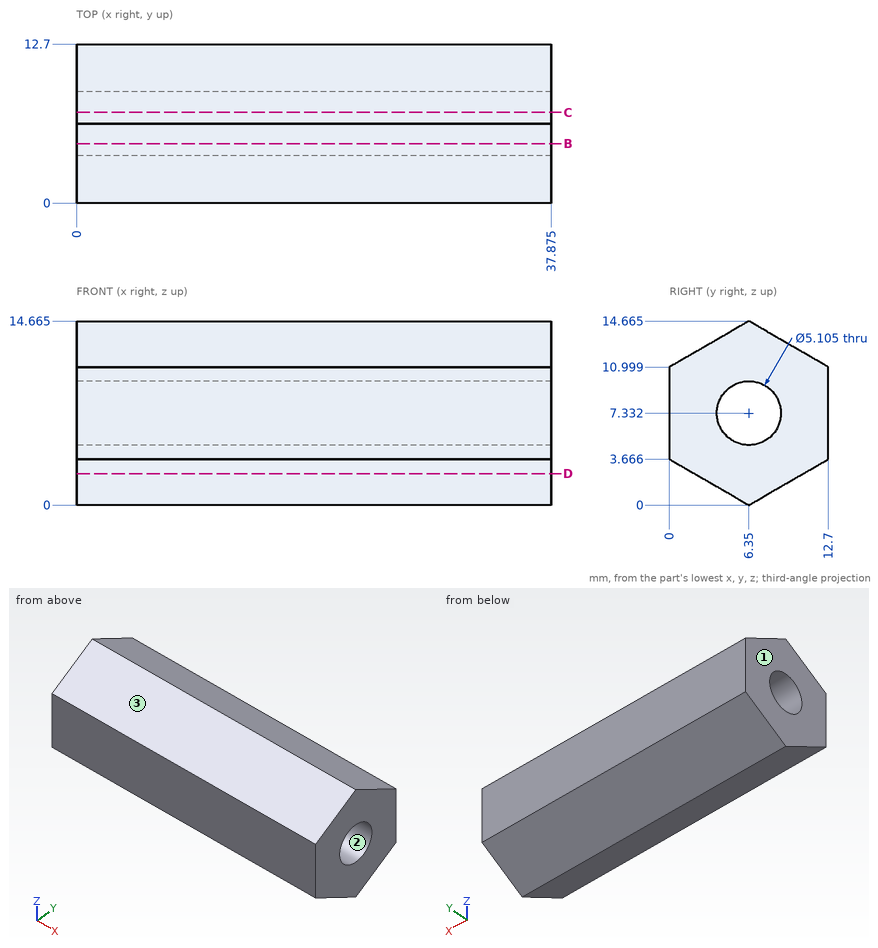
Design review of the part shown in the three views and the two pictorial views. Dimensions are in mm from the part's minimum x, y and z. Give positions to 0.01 mm unless a question says otherwise; leave off trailing zeros. Write each loop counter-clockwise with the first axis right and the second up, starting at its lowest first coordinate (ties: lowest second). Pieces come first, ordered by that corner, then holes. Notation, with made-up numbers: M 28,55 L 73,55 A17 cw 73,60 Z; hole C 38,68.25 d9. An arc over 180 degrees is marked long. Return JSON: item names as keys, results as strings. Group by question number.
Item 1: Wall thickness on line 1 along Z through (x, y) = (15, 7) (1 decimal); line 2 along Y through (x, z) = (25.5, 6.75) (1 decimal); line 3 along Z through (x, y) = (28, 5.25) (1 decimal): over which ranges is each line inside the solid? List them lowest first.
Item 2: The part is to be moulded in two halves that separate along Z. For the marked faces 1, 2 and 3, say which applies: pulls with the +Z half, pulls with the -Z half, needs draft (parallel to the pull), parting line crosses it, or undercut.
Item 3: Take a section at B-B (y = 4.75). Give the boundary of the cut face in (x, z) (1 decimal).
Item 4: Take a section at D-D (z = 2.5). Give the boundary of the cut face in (x, y) (1 decimal), plus the area to 3 significant figures.
Item 5: Take a section at C-C (y = 7.25). Give the boundary of the cut face in (x, z) (1 decimal).
Item 6: Clearance check with flat-ended pins moving along their axes: pin 1 Ø4 at (x, z) = (10.5, 4) entering from -Y; pin 2 Ø4 at (y, z) = (6, 7.5) entering from +X; pin 3 Ø3 at (x, z) = (31.5, 1.5) entering from +Y (1 decimal); pin 4 Ø6 at (x, y) = (9.5, 10) entering from +Z. State where each tip first meets the part, or that it passes through.
Return value:
{
 "1": {"line 1": "z = 0.4 to 4.9, 9.8 to 14.3", "line 2": "y = 0 to 3.9, 8.8 to 12.7", "line 3": "z = 0.6 to 5, 9.6 to 14"},
 "2": {"face 1": "needs draft", "face 2": "undercut", "face 3": "pulls with the +Z half"},
 "3": {"outline": "M 0,0.9 L 37.9,0.9 L 37.9,5.3 L 0,5.3 Z; M 0,9.3 L 37.9,9.3 L 37.9,13.7 L 0,13.7 Z"},
 "4": {"outline": "M 0,2 L 37.9,2 L 37.9,10.7 L 0,10.7 Z", "area": "328 mm2"},
 "5": {"outline": "M 0,0.5 L 37.9,0.5 L 37.9,4.9 L 0,4.9 Z; M 0,9.7 L 37.9,9.7 L 37.9,14.1 L 0,14.1 Z"},
 "6": {"pin 1": "stops at y = 0", "pin 2": "passes through", "pin 3": "stops at y = 11.5", "pin 4": "stops at z = 14.29"}
}
